Source: CAD feature listing. Evaluate the final solid. Frame: model axes, mm. A direction names the side the tool comes from. Coordinates: 2 decimals unless noted, no trailing zeros. Write each loop counter-clockwise with the first axis right and the second up, starting at its lowest first coordinate (ties: lowest second). Pieces come first, ordered by that corner, then holes. Notation, with made-up numbers: M 40,41 L 69,41 A35 cw 69,77 Z; hole C 32.25,63 d2. An arc over 180 degrees is marked long. Answer as CSV lines item,"result". Start each with the question number.
1. Section C-C on y = -35. Return the cut outline in (x, z), plus the area to 3 significant figures.
2. Reachability of faces 4 (the face through (-42, -50, 25)), 5 (the face through (3, -20, 24)) from +Z, -Z, +X, -X, +Y, -Y: full face, straight path, thin tool, end or side. Return the list, or none.
3. Mould query, pull axis X, two halves, no side actions, for faces 1 (the face through (40.456, -35, 16)), 2 (the face through (34.237, -19.094, 35.276)), 3 (the face through (51, -50, 13)). Classes: pulls with the +X half, pulls with the -X half, needs draft (parallel to the pull), parting line crosses it, or undercut.
4. Section D-D on y = -10.5. Return the cut outline in (x, z).
5. Section B-B on z = 11. Return the cut outline in (x, y), plus the area to 3 significant figures.
6. Contact query for flat-ended pins moving along their axis: pin 1 Ø1 at (y, z) = (-8, 44) entering from +X; pin 2 Ø4 at (x, z) = (-29.5, 11.5) entering from -Y; pin 3 Ø3 at (x, y) = (39.5, -22) entering from +Z. Output: stop coordinate, or through.
7. Section A-A on y = -45.5. Return the cut outline in (x, z).
8. Line query: probe 1 along X at (y, z) = (-39.5, 3.5); probe 2 along Y at (x, z) = (24.5, 13); probe 3 along X at (y, z) = (-24, 41). Output: solid intervals per line, ascending. Write a range as [from, to].
```python
from build123d import *

# Parameters (mm, degrees)
F0_W     = 110
F0_H     = 60
F1_DEPTH = 50
F2_W     = 74.486891
F2_H     = 60
F3_DEPTH = 30
F5_DEPTH = 15
F7_DEPTH = 50


with BuildPart() as f1:
    # F0 (on Front) → F1 (new body)
    with BuildSketch(Plane.XZ):
        with Locations((5.968994, 30)):
            Rectangle(F0_W, F0_H)
    extrude(amount=F1_DEPTH)

    # F2 (on face) → F3 (cut)
    with BuildSketch(Plane.XZ.offset(50)):
        with Locations((3.212439, 30)):
            Rectangle(F2_W, F2_H)
    extrude(amount=-F3_DEPTH, mode=Mode.SUBTRACT)

    # F4 (on face) → F5 (cut)
    with BuildSketch(Plane(origin=(-49.031006, 0, 0), x_dir=(0, -1, 0), z_dir=(-1, 0, 0))):
        Polygon((50, 60), (30, 60), (50, 50), align=None)
    extrude(amount=-F5_DEPTH, mode=Mode.SUBTRACT)

    # F6 (on face) → F7 (cut)
    with BuildSketch(Plane(origin=(0, 0, 0), x_dir=(-1, 0, 0), z_dir=(0, 1, 0))):
        Polygon((-60.968994, 20), (9.031006, 60), (-60.968994, 60), align=None)
    extrude(amount=-F7_DEPTH, mode=Mode.SUBTRACT)


solid = f1.part
```
Values:
1,outline,"M -49.03,0 L -34.03,0 L -34.03,57.5 L -49.03,57.5 Z; M 40.46,0 L 60.97,0 L 60.97,20 L 40.46,31.72 Z"
1,area,"1,390 mm²"
2,face 4,"+Z, -Z, +X, -X, -Y"
2,face 5,"+Z, -Z, -Y"
3,face 1,"undercut"
3,face 2,"pulls with the +X half"
3,face 3,"needs draft"
4,outline,"M -49.03,0 L 60.97,0 L 60.97,20 L -9.03,60 L -49.03,60 Z"
5,outline,"M -49.03,-50 L -34.03,-50 L -34.03,-20 L 40.46,-20 L 40.46,-50 L 60.97,-50 L 60.97,0 L -49.03,0 Z"
5,area,"3,270 mm²"
6,pin 1,"x = 19.84"
6,pin 2,"y = -20"
6,pin 3,"z = 31.72"
7,outline,"M -49.03,0 L -34.03,0 L -34.03,52.25 L -49.03,52.25 Z; M 40.46,0 L 60.97,0 L 60.97,20 L 40.46,31.72 Z"
8,probe 1,"[-49.03, -34.03], [40.46, 60.97]"
8,probe 2,"[-20, 0]"
8,probe 3,"[-49.03, -34.03]"
